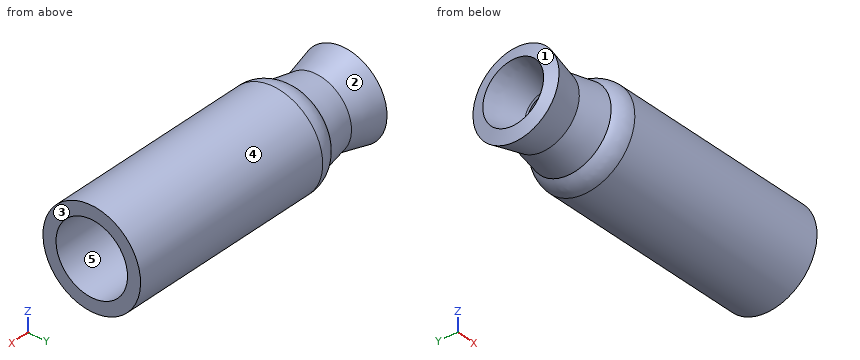
```python
from build123d import *


with BuildPart() as part:
    # Sketch1 → Revolve1 (revolve)
    with BuildSketch(Plane.XY, mode=Mode.PRIVATE) as revolve1_sk:
        with BuildLine():
            Line((52.322643444, 27.400944548), (-107.862323025, 27.400944548))
            ThreePointArc((-107.862323025, 27.400944548), (-111.689157349, 26.639739873), (-114.933390837, 24.47201236))
            Line((-114.933390837, 24.47201236), (-143.633390837, 18.950120538))
            Line((-143.633390837, 18.950120538), (-143.633390837, 14.210120538))
            Line((-143.633390837, 14.210120538), (-144.933390837, 14.7))
            add(Edge.make_bspline(
                [(-171.933390837, 23.283456642), (-158.435473315, 19.858823042), (-144.933390837, 14.7)],
                knots=[0, 0, 0, 1, 1, 1], degree=2))
            Line((-171.933390837, 23.283456642), (-169.474152094, 32.976348099))
            Line((-169.474152094, 32.976348099), (-144.933390837, 27.131544172))
            Line((-144.933390837, 27.131544172), (-122.004458649, 31.543080172))
            ThreePointArc((-122.004458649, 31.543080172), (-115.515991673, 35.878535198), (-107.862323025, 37.400944548))
            Line((-107.862323025, 37.400944548), (52.322643444, 37.400944548))
            Line((52.322643444, 37.400944548), (52.322643444, 27.400944548))
        make_face()
    revolve(revolve1_sk.sketch.rotate(Axis((0, 0, 0), (-1, 0, 0)), 90), axis=Axis((0, 0, 0), (-1, 0, 0)))


solid = part.part
```
Model file for the job. Use its own axes, mm. Face numbers are marked on the shaded views. A direction names the side the tool comes from. Coordinates: 2 decimals unless noted, no trailing zeros. Loops run counter-clockwise (first coordinate to the right, second up) from the corner with the lowest first, then second, coordinate; pieces in that order, holes last. Notation, with made-up numbers: (75, -27.5) - (81, -27.5) arc R21 ccw to (81, -22.5) - close; hole circle Ø1 at (-26.5, -22.5). An arc over 180 degrees is marked (long way). Answer as a JSON object with one key per item and string values. Group by question number.
(1) Tool access for the marked faces 1 and 2: list every direction of +Z, -Z, +X, -X, +Y, -Y with a clear straight run to the whole face (end or side of a thin tool).
(2) Cut at B-B (x = -88.5). Give the cut face in (y, z), then the cut area to 3 significant figures.
(3) Flat gauge pins, fed straight in: pin 1 (1.5 mm diameter, centred on x = -24, z = -6, fed in from +Y); pin 2 (5 mm diameter, centred on x = -28.5, y = -9, fed in from -Z); pin 3 (3 mm diameter, centred on y = -21, z = 12.5, fed in from +X). Where does each tip first touch, or does it go through?
(4) Two-plate mould, pull along Z, no slides. Class the marked faces 3, 4 and 5: released by +Z, released by -Z, zero draft, split by the parting line, or undercut.
(5) Probe line 1 along Y through (x, z) = (-13, 0); line 2 along Y through (x, z) = (-30.5, -20); line 3 along Z through (x, y) = (-69.5, -9.5). List the from-to ranges inside material, lowest first.
(6) Cut at A-A (x = -139). Give the cut face in (y, z).
Geometry says:
{
 "1": {"face 1": "-X", "face 2": "none"},
 "2": {"outline": "circle Ø74.8 at (0, 0); hole circle Ø54.8 at (0, 0)", "area": "2,040 mm^2"},
 "3": {"pin 1": "stops at y = 37.03", "pin 2": "stops at z = -36.83", "pin 3": "stops at x = -113.07"},
 "4": {"face 3": "zero draft", "face 4": "split by the parting line", "face 5": "undercut"},
 "5": {"line 1": "y = -37.4 to -27.4, 27.4 to 37.4", "line 2": "y = -31.6 to -18.73, 18.73 to 31.6", "line 3": "z = -36.17 to -25.7, 25.7 to 36.17"},
 "6": {"outline": "circle Ø56.55 at (0, 0); hole circle Ø39.68 at (0, 0)"}
}
